Model file for the job. Use its own axes, mm. Give positions to 0.01 mm unless a question says otherwise; leave off trailing zeros. Order: outer loops, then holes, each group sorted by start corner. A loop starts at its lowest first (then second) coordinate and runs counter-clockwise, first axis right, second up. Notation, with made-up numbers: M 49.5,-16.5 L 106.5,-16.5 A10 ccw 106.5,-1.5 Z; hole C 16.25,21 d8. An arc over 180 degrees is marked long. Return JSON: item names as keys, results as strings. Group by question number.
1. Slice it at A-A on z = -50.8. List the corners of the cut face in (x, y) (3 decimals).
2. Slice it at D-D on x = 93. List the corners of the cut face in (y, z), then the cut area to 3 significant figures.
3. Slice it at C-C on y = 5. List the corners of the cut face in (x, z) (3 decimals).
4. Slice it at B-B on x = 50.8. List the corners of the cut face in (y, z) (3 decimals).
5. Wall check: probe 1 along Z at (x, y) = (92, 2.75); probe 2 along X at (y, z) = (0.5, -92); probe 3 along Z at (x, y) = (97, 1.75). Give the ranges that are in metal, low to high. Write a range as [from, to].
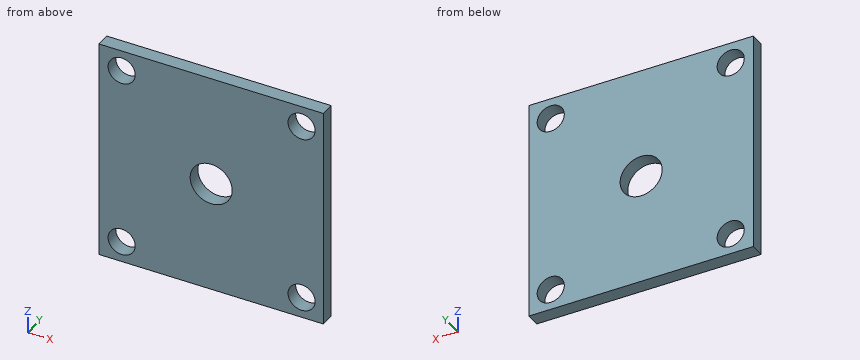
from build123d import *

# Parameters (mm, degrees)
SKETCH1_W                   = 101.6
SKETCH1_H                   = 101.6
BOSS_EXTRUDE1_DEPTH         = 6.35
F_9_16_12_TAPPED_HOLE1_D    = 12.30376
F_3_4_0_75_DIAMETER_HOLE1_D = 19.05


with BuildPart() as part:
    # Sketch1 → Boss-Extrude1 (new body)
    with BuildSketch(Plane(origin=(0, 0, 0), x_dir=(1, 0, 0), z_dir=(0, 1, 0))):
        with Locations((50.8, 50.8)):
            Rectangle(SKETCH1_W, SKETCH1_H)
    extrude(amount=BOSS_EXTRUDE1_DEPTH)

    # 9/16-12 Tapped Hole1 (through all)
    with Locations(Plane(origin=(0, 6.35, 0), x_dir=(1, 0, 0), z_dir=(0, 1, 0))):
        with Locations((10.266147992, 92.075), (91.751726771, 9.525), (91.751726771, 92.075), (10.266147992, 9.525)):
            Hole(F_9_16_12_TAPPED_HOLE1_D / 2)

    # 3/4 (0.75) Diameter Hole1 (through all)
    with Locations(Plane(origin=(0, 6.35, 0), x_dir=(1, 0, 0), z_dir=(0, 1, 0))):
        with Locations((50.8, 50.8)):
            Hole(F_3_4_0_75_DIAMETER_HOLE1_D / 2)


solid = part.part
Result:
{
 "1": {"outline": "M 0,0 L 41.275,0 L 41.275,6.35 L 0,6.35 Z; M 60.325,0 L 101.6,0 L 101.6,6.35 L 60.325,6.35 Z"},
 "2": {"outline": "M 0,-101.6 L 6.35,-101.6 L 6.35,-98.1 L 0,-98.1 Z; M 0,-86.05 L 6.35,-86.05 L 6.35,-15.55 L 0,-15.55 Z; M 0,-3.5 L 6.35,-3.5 L 6.35,0 L 0,0 Z", "area": "492 mm2"},
 "3": {"outline": "M 0,-101.6 L 101.6,-101.6 L 101.6,0 L 0,0 Z; hole C 10.266,-92.075 d12.304; hole C 10.266,-9.525 d12.304; hole C 50.8,-50.8 d19.05; hole C 91.752,-92.075 d12.304; hole C 91.752,-9.525 d12.304"},
 "4": {"outline": "M 0,-101.6 L 6.35,-101.6 L 6.35,-60.325 L 0,-60.325 Z; M 0,-41.275 L 6.35,-41.275 L 6.35,0 L 0,0 Z"},
 "5": {"probe 1": "z = [-101.6, -98.22], [-85.93, -15.67], [-3.38, 0]", "probe 2": "x = [0, 4.11], [16.42, 85.6], [97.9, 101.6]", "probe 3": "z = [-101.6, -95.28], [-88.87, -12.73], [-6.32, 0]"}
}
